Build history of the part. All positions in model axes, mm. A direction names the side the tool comes from. Coordinates: 2 decimals unless noted, no trailing zeros. Loops run counter-clockwise (first coordinate to the right, second up) from the corner with the lowest first, then second, coordinate; pieces in that order, holes last.
Item 1: Cut at D-D (y = 44). List the corners of the cut face in (x, z).
Item 2: Cut at C-C (x = -18.5). List the corners of the cut face in (y, z), and give its area (3 significant figures).
Item 3: Drill centre lines: line 1 along Z through (x, y) = (17.5, 12); line 2 along Y through (x, z) = (-16.5, 28); line 3 along X through (y, z) = (51, 34). Where is each one in solid material? Low to high.
Item 4: Flat gauge pins, fed straight in: pin 1 (12 mm diameter, centred on x = 2, y = -15.5, fed in from -Z); pin 2 (12 mm diameter, centred on x = -17, y = 31, fed in from +Z); pin 3 (7.5 mm diameter, centred on x = 3.5, z = 28.5, fed in from -Y). Where does each tip first touch, or does it go through?
Item 5: Cut at A-A (y = -12). List the corners of the cut face in (x, z), and give its area (3 significant figures).
Item 6: Mould opens along X. For faces 1 (the face through (17, 50, 44.45)), 2 (the face through (-14.303, -30, 9)), 3 (the face through (17.68, -42.11, 9.39)) say: released by +X, released by -X, zero draft, split by the parting line, or undercut.
Item 7: Cut at B-B (z = 38.5). List the corners of the cut face in (x, y).
Item 8: 3-axis set-ups, long thin cutter, end or side, ignore diameter. For faces 4 (the face through (-7, 1, 19.05)), 5 (the face through (-23.955, 50.006, 31.543)), 6 (the face through (1.572, -29, 9)): which of +Z, -Z, +X, -X, +Y, -Y reach the whole face in a straight line?
from build123d import *

# Parameters (mm, degrees)
F1_DEPTH = 19.05
F0_W     = 28.575
F0_H     = 25.4
F2_DEPTH = 31.75
F0_W_2   = 19.05
F3_DEPTH = 44.45
F5_DEPTH = 25.401


with BuildPart() as f1:
    # F0 (on Top) → F1 (new body)
    with BuildSketch(Plane.XY):
        Polygon((-20.6530114731, 37.4838656797), (-39.7030114731, 37.4838656797), (-39.7030114731, -26.0161343203), (-21.3721404263, -57.7661343203), (-14.3030114731, -57.7661343203), (-14.3030114731, -0.6161343203), (1.5719885269, -0.6161343203), (1.5719885269, -57.7661343203), (8.6411174801, -57.7661343203), (26.9719885269, -26.0161343203), (26.9719885269, 37.4838656797), (7.9219885269, 37.4838656797), align=None)
    extrude(amount=F1_DEPTH)

    # F0 (on Top) → F2 (join)
    with BuildSketch(Plane.XY):
        with Locations((-6.3655114731, 50.1838656797)):
            Rectangle(F0_W, F0_H)
    extrude(amount=F2_DEPTH)

    # F0 (on Top) → F3 (join)
    with BuildSketch(Plane.XY):
        with Locations((-30.1780114731, 50.1838656797)):
            Rectangle(F0_W_2, F0_H)
        with Locations((17.4469885269, 50.1838656797)):
            Rectangle(F0_W_2, F0_H)
    extrude(amount=F3_DEPTH)

    # F4 (on face) → F5 (cut, through all)
    with BuildSketch(Plane.XZ.offset(-37.4838656797)):
        Polygon((-20.6530114731, 31.75), (-20.6530114731, 44.45), (-27.1653852305, 31.342598024), align=None)
        Polygon((7.9219885269, 44.45), (7.9219885269, 31.75), (15.2543369456, 31.75), align=None)
    extrude(amount=-F5_DEPTH, mode=Mode.SUBTRACT)


solid = f1.part
Filled sheet:
1. outline: (-39.7, 0) - (26.97, 0) - (26.97, 44.45) - (7.92, 44.45) - (15.25, 31.75) - (-20.65, 31.75) - (-27.17, 31.34) - (-20.65, 44.45) - (-39.7, 44.45) - close
2. outline: (-57.77, 0) - (62.88, 0) - (62.88, 31.75) - (37.48, 31.75) - (37.48, 19.05) - (-57.77, 19.05) - close
2. area: 2,620 mm2
3. line 1: z = 0 to 19.05
3. line 2: y = 37.48 to 62.88
3. line 3: x = -39.7 to -25.85, 13.96 to 26.97
4. pin 1: stops at z = 0
4. pin 2: stops at z = 19.05
4. pin 3: stops at y = 37.48
5. outline: (-39.7, 0) - (-14.3, 0) - (-14.3, 19.05) - (-39.7, 19.05) - close; (1.57, 0) - (26.97, 0) - (26.97, 19.05) - (1.57, 19.05) - close
5. area: 968 mm2
6. face 1: zero draft
6. face 2: undercut
6. face 3: released by +X
7. outline: (-39.7, 37.48) - (-23.61, 37.48) - (-23.61, 62.88) - (-39.7, 62.88) - close; (11.36, 37.48) - (26.97, 37.48) - (26.97, 62.88) - (11.36, 62.88) - close
8. face 4: +Z, +X, -X, -Y
8. face 5: +Y, -Y
8. face 6: +Z, -Z, -Y
